Part model, mm, in its own coordinate system. Round coordinates to 2 decimals unless told otherwise and drop trailing zeros. Write each loop counter-clockwise with the first axis right and the second up, starting at its lowest first coordinate (ties: lowest second). Pieces come first, ordered by that corner, then holes. Notation, with made-up numbers: (59, 40) -> (74, 40) arc R22 cw to (74, 60) -> close; hole circle Ø11 at (15, 20.25). An arc over 180 degrees is marked (long way). Return JSON: item names as keys, results as strings. Group by question number.
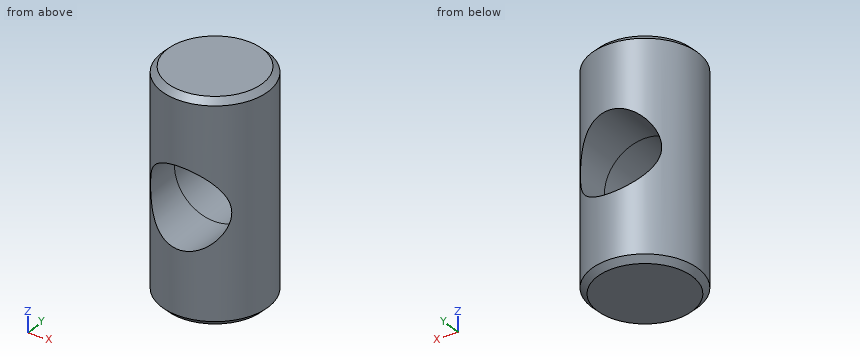
```python
from build123d import *

# Parameters (mm, degrees)
SKETCH1_R               = 4.65
BOSS_EXTRUDE1_DEPTH     = 19.1
SKETCH2_R               = 3.5
CUT_EXTRUDE1_DEPTH      = 5.65
CUT_EXTRUDE1_DEPTH_BACK = 5.65
CHAMFER1_SIZE           = 0.5


with BuildPart() as part:
    # Sketch1 → Boss-Extrude1 (new body)
    with BuildSketch(Plane.XY):
        Circle(SKETCH1_R)
    extrude(amount=BOSS_EXTRUDE1_DEPTH)

    # Sketch2 → Cut-Extrude1 (cut, two sides)
    with BuildSketch(Plane(origin=(0, 0, 0), x_dir=(1, 0, 0), z_dir=(0, 1, 0))) as cut_extrude1_sk:
        with Locations((0, -9.55)):
            Circle(SKETCH2_R)
    extrude(amount=CUT_EXTRUDE1_DEPTH, mode=Mode.SUBTRACT)
    extrude(cut_extrude1_sk.sketch, amount=-CUT_EXTRUDE1_DEPTH_BACK, mode=Mode.SUBTRACT)

    # Chamfer1
    chamfer1_edges = [part.edges().sort_by_distance(p)[0] for p in [
        (-4.65, 0, 0),
        (-4.65, 0, 19.1),
    ]]
    chamfer(chamfer1_edges, length=CHAMFER1_SIZE)


solid = part.part
```
Item 1: Cut at A-A (x = 0). Write the cut outline in (y, z).
Item 2: Flat gauge pin, fed straight in: P1, Ø2, axis at y = 2, z = 13.5, coming from the +X side. Where does the tip first touch, or does it go through?
Item 3: Cut at B-B (z = 9.55). Write the cut outline in (x, y).
Item 4: Cut at C-C (z = 13.5). Write the cut outline in (x, y), then the cut area to 3 significant figures.
Item 5: Wall check: L1, parallel to Z at x = 0, y = 2.4; L2, parallel to Z at x = 2, y = -2; L3, parallel to X at y = 1.75, z = 9.55. Give the ranges that are in metal, low to high.
Checks:
{
 "1": {"outline": "(-4.65, 0.5) -> (-4.15, 0) -> (4.15, 0) -> (4.65, 0.5) -> (4.65, 6.05) -> (-4.65, 6.05) -> close; (-4.65, 13.05) -> (4.65, 13.05) -> (4.65, 18.6) -> (4.15, 19.1) -> (-4.15, 19.1) -> (-4.65, 18.6) -> close"},
 "2": {"P1": "stops at x = 4.54"},
 "3": {"outline": "(-3.5, -3.06) -> (-3.5, 3.06) arc R4.65 ccw to start; (3.5, -3.06) arc R4.65 ccw to (3.5, 3.06) -> close"},
 "4": {"outline": "circle Ø9.3 at (0, 0)", "area": "67.9 mm2"},
 "5": {"L1": "z = 0 to 6.05, 13.05 to 19.1", "L2": "z = 0 to 6.68, 12.42 to 19.1", "L3": "x = -4.31 to -3.5, 3.5 to 4.31"}
}
